Autodesk Inventor part; units mm, degrees
ref_plane "YZ Plane" through (0, 0, 0) normal (1, 0, 0) x (0, 1, 0)
ref_plane "XZ Plane" through (0, 0, 0) normal (0, 1, 0) x (-1, 0, 0)
ref_plane "XY Plane" through (0, 0, 0) normal (0, 0, 1) x (1, 0, 0)
sketch "Sketch1" plane through (0, 0, 0) normal (1, 0, 0) x (0, 1, 0)
  line L0 (0, 0) -> (28.5, 0)
  line L1 (24.95, 1.5) -> (4.5855, 1.5)
  line L2 (2.8178, 2.2322) -> (0.3, 4.75)
  line L3 (0.3, 4.75) -> (0, 4.75)
  line L4 (0, 4.75) -> (0, 0)
  arc A0 (28.5, 0) -> (27, 1.5) centre (27, 0) ccw
  line L5 (24.95, 1.5) -> (24.95, 1.15)
  line L6 (24.95, 1.15) -> (25.6, 1.15)
  line L7 (25.6, 1.15) -> (25.6, 1.5)
  line L8 (25.6, 1.5) -> (27, 1.5)
  arc A1 (2.8178, 2.2322) -> (4.5855, 1.5) centre (4.5855, 4) ccw
  dimension "d1" = 4.75
  dimension "d2" = 1.5
  dimension "d3" = 0.3
  dimension "d4" = 45
  dimension "d5" = 1.5
  dimension "d6" = 1.15
  dimension "d8" = 0.65
  dimension "d9" = 1.4
  dimension "d10" = 27
  dimension "d11" = 2.5
revolve "Revolution1" add sketch "Sketch1" angle 360 about axis through (0, 0, 0) along (0, 1, 0)
properties part number "Component 24 (Valve)"
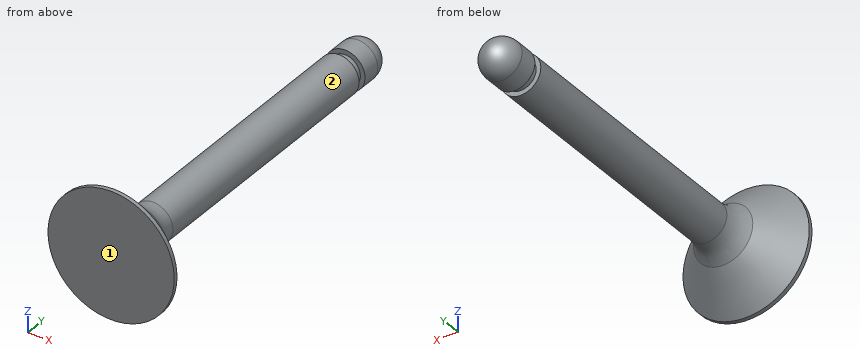
Design review of the part built by this model. Coordinates are the model's own, in mm. Face numbers are marked on the shaded views. A direction names the side the tool comes from. Give positions to 0.01 mm unless a question says otherwise; leave off trailing zeros. Write each loop counter-clockwise with the first axis right and the second up, starting at its lowest first coordinate (ties: lowest second). Pieces come first, ordered by that corner, then holes. Notation, with made-up numbers: M -17,-34.75 L 8,-34.75 A18 cw 8,-25.75 Z; hole C -24.5,12.25 d9. An arc over 180 degrees is marked long. Answer as a JSON object with one key per item and string values. Group by question number.
1) Clearance check with flat-ended pins moving along their axes: pin 1 Ø5 at (x, y) = (-2, 23) entering from -Z; pin 2 Ø1.5 at (y, z) = (24.5, -3) entering from -X; pin 3 Ø4 at (y, z) = (25, 0.5) entering from -X; pin 4 Ø2 at (x, y) = (-2, 12) entering from +Z. State where each tip first meets the part, or that it passes through.
2) We need section A-A (z = 0). Give the boundary of the cut face in (x, y).
3) For line 1 along Y through (x, z) = (0, 1.25); line 2 along Y through (x, z) = (0.25, -2.5); line 3 along X through (y, z) = (13, -0.75), list the stretches that pass through material, from the lowest coordinate up.
4) We need section B-B (x = 0). Give the boundary of the cut face in (y, z), and give its area (3 significant figures).
5) We need section C-C (y = 10.5). Give the boundary of the cut face in (x, z), and give its area (3 significant figures).
6) Tool access review of the marked faces 1 and 2: name each direction out of +Z, -Z, +X, -X, +Y, -Y from which nothing blocks a thin tool from reaching the whole face with its end or side.
Answer key:
{
 "1": {"pin 1": "stops at z = -1.5", "pin 2": "passes through", "pin 3": "stops at x = -1.5", "pin 4": "stops at z = 1.12"},
 "2": {"outline": "M -4.75,0 L 4.75,0 L 4.75,0.3 L 2.23,2.82 A2.5 cw 1.5,4.59 L 1.5,24.95 L 1.15,24.95 L 1.15,25.6 L 1.5,25.6 L 1.5,27 A1.5 ccw -1.5,27 L -1.5,25.6 L -1.15,25.6 L -1.15,24.95 L -1.5,24.95 L -1.5,4.59 A2.5 cw -2.23,2.82 L -4.75,0.3 Z"},
 "3": {"line 1": "y = 0 to 24.95, 25.6 to 27.83", "line 2": "y = 0 to 2.54", "line 3": "x = -1.3 to 1.3"},
 "4": {"outline": "M 0,-4.75 L 0.3,-4.75 L 2.82,-2.23 A2.5 cw 4.59,-1.5 L 24.95,-1.5 L 24.95,-1.15 L 25.6,-1.15 L 25.6,-1.5 L 27,-1.5 A1.5 ccw 27,1.5 L 25.6,1.5 L 25.6,1.15 L 24.95,1.15 L 24.95,1.5 L 4.59,1.5 A2.5 cw 2.82,2.23 L 0.3,4.75 L 0,4.75 Z", "area": "96.9 mm²"},
 "5": {"outline": "C 0,0 d3", "area": "7.07 mm²"},
 "6": {"face 1": "+Z, -Z, +X, -X, -Y", "face 2": "+Y"}
}
